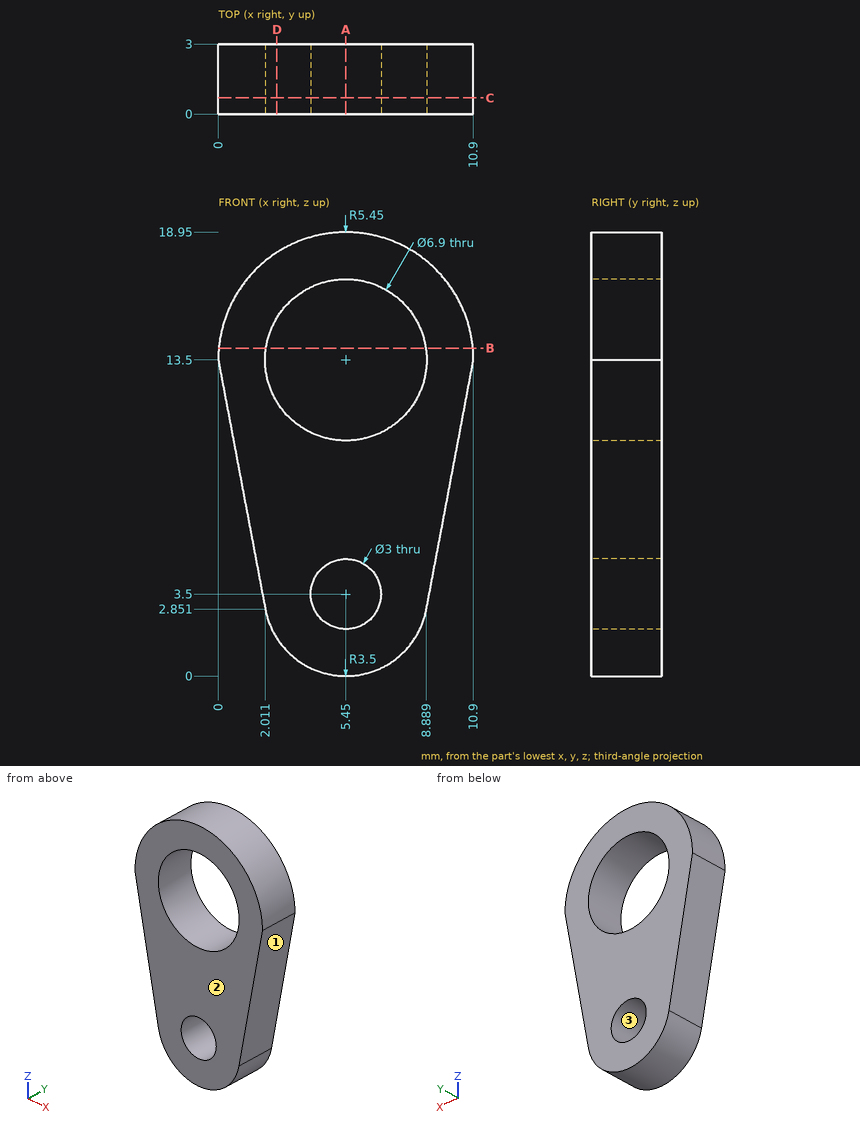
Drawing for the job (mm, zero at the part's lowest x, y, z). Give positions to 0.01 mm unless a question says otherwise; leave off trailing zeros. Order: outer loops, then holes, each group sorted by start corner. A loop starts at its lowest first (then second) coordinate and runs counter-clockwise, first axis right, second up. Notation, with made-up numbers: (47.25, -3.75) - (71.25, -3.75) arc R21 cw to (71.25, 5.25) - close; hole circle Ø11 at (41, 6). An arc over 180 degrees is marked (long way). Use one line per item in the form item = value.
Item 1: Slice it at A-A on x = 5.45. Give the cut face in (y, z).
Solution:
outline = (0, 0) - (3, 0) - (3, 2) - (0, 2) - close; (0, 5) - (3, 5) - (3, 10.05) - (0, 10.05) - close; (0, 16.95) - (3, 16.95) - (3, 18.95) - (0, 18.95) - close
Item 2: Slice it at C-C on y = 0.7. Give the cut face in (x, z), and give its area (3 significant figures).
Solution:
outline = (0, 13.5) - (2.01, 2.85) arc R3.5 ccw to (8.89, 2.85) - (10.9, 13.5) arc R5.45 ccw to start; hole circle Ø6.9 at (5.45, 13.5); hole circle Ø3 at (5.45, 3.5)
area = 112 mm2
Item 3: Pin check, flat tip, straight feed: pin 1 Ø2.5 at (x, z) = (5.45, 3.5) entering from +Y. Stop position of the tip, or through.
Solution:
pin_1 = through
Item 4: Slice it at B-B on z = 14. Give the cut face in (x, y), and give its area (3 significant figures).
Solution:
outline = (0.02, 0) - (2.04, 0) - (2.04, 3) - (0.02, 3) - close; (8.86, 0) - (10.88, 0) - (10.88, 3) - (8.86, 3) - close
area = 12.1 mm2
Item 5: Two-plate mould, pull along X, no slides. Class the marked faces 1, 2 and 3: released by +X, released by -X, zero draft, split by the parting line, or undercut.
Solution:
face_1 = released by +X
face_2 = zero draft
face_3 = undercut
Item 6: Probe probe 1 along Z at (x, y) = (5.45, 1); probe 2 along Z at (x, y) = (6.25, 1.95) (1 decimal); probe 3 along X at (y, z) = (2.05, 13.5). List the from-to ranges inside material, lowest first. Write a range as from..to.
Solution:
probe_1 = 0..2, 5..10.05, 16.95..18.95
probe_2 = 0.1..2.2, 4.8..10.1, 16.9..18.9
probe_3 = 0..2, 8.9..10.9
Item 7: Slice it at D-D on x = 2.5. Give the cut face in (y, z).
Solution:
outline = (0, 1.62) - (3, 1.62) - (3, 11.71) - (0, 11.71) - close; (0, 15.29) - (3, 15.29) - (3, 18.08) - (0, 18.08) - close
